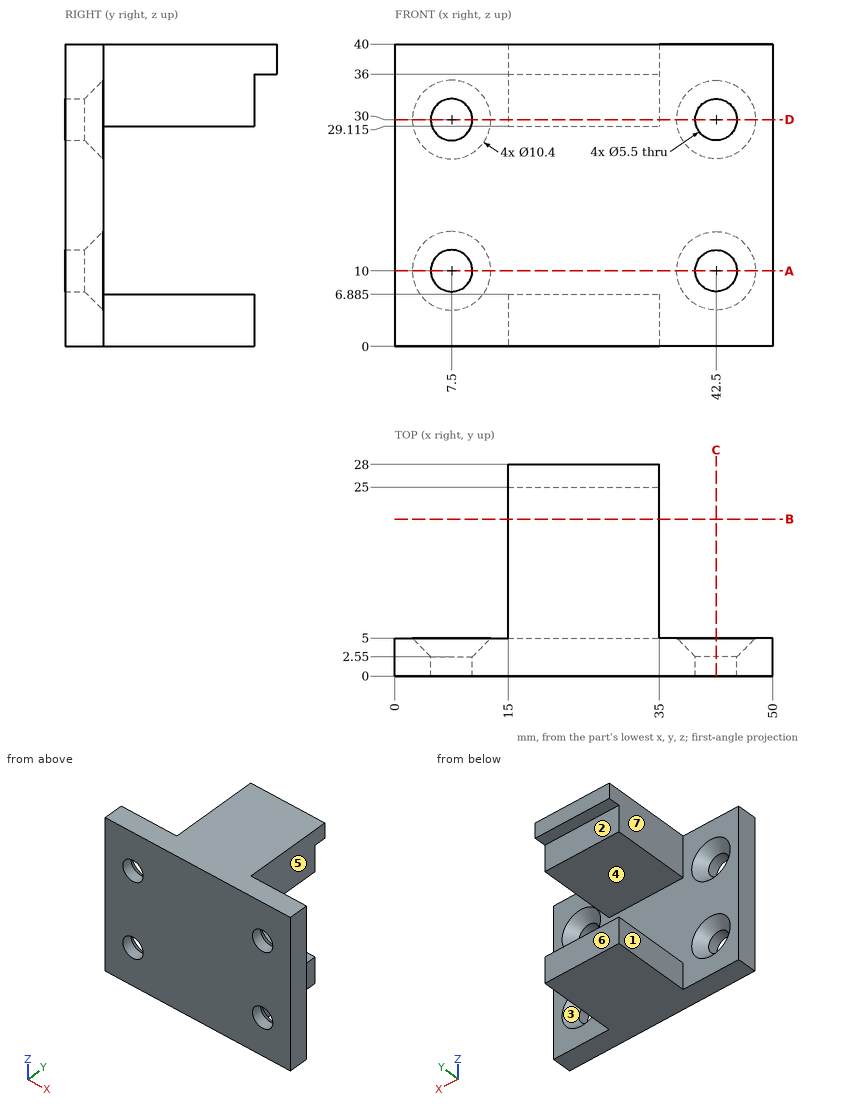
The figure shows three views and two pictorial views of one solid part (mm, origin at its lowest corner). Answer the questions. A direction names the side the tool comes from. Give positions to 0.01 mm unless a question says otherwise; leave off trailing zeros. Loops run counter-clockwise (first coordinate to the right, second up) from the corner with the lowest first, then second, coordinate; pieces in that order, holes last. Notation, with made-up numbers: (83.5, -16) -> (91.5, -16) arc R10 ccw to (91.5, -4) -> close; hole circle Ø8 at (40.5, 45.5). An arc over 180 degrees is marked (long way). Use a Markdown table: item, result. Add a question column.
1. Section C-C on x = 42.5 is taken. Determine the outline of the cut face in (y, z).
2. Section B-B on y = 20.75 is taken. Determine the outline of the cut face in (x, z) (3 decimals), and give its area (3 significant figures).
3. Find the intervals of material crossed by probe 1 along X at (y, z) = (1.45, 10); probe 2 along Z at (x, y) = (32, 14.5) (3 decimals); probe 3 along Z at (x, y) = (7.5, 1.4), in increasing order.
4. Section D-D on z = 30 is taken. Determine the outline of the cut face in (x, y), and give its area (3 significant figures).
5. Flat-ended cylindrical pins translate along their axes: pin 1 Ø10 at (x, y) = (9.5, 22) entering from -Z; pin 2 Ø7.5 at (y, z) = (16.5, 3.5) entering from -X; pin 3 Ø9 at (x, z) = (7.5, 30) entering from +Y; pin 4 Ø2 at (x, z) = (21, 31) entering from +Y. Find the tip coordinate at first contact, or state that the pin passes through.
6. For the marked faces 4, 5, 6 and 7, determine the directions among +Z, -Z, +X, -X, +Y, -Y from which every point of the face is accessible in a straight line to the end or side of a thin tool.
7. Determine the mould class of the marked faces 1, 2 and 3 for opening direction X: released by +X, released by -X, zero draft, split by the parting line, or undercut.
8. Section A-A on z = 10 is taken. Determine the outline of the cut face in (x, y), and give its area (3 significant figures).
Results below:
| question | item | result |
|---|---|---|
| 1 | outline | (0, 0) -> (5, 0) -> (5, 4.8) -> (2.55, 7.25) -> (0, 7.25) -> close; (0, 12.75) -> (2.55, 12.75) -> (5, 15.2) -> (5, 24.8) -> (2.55, 27.25) -> (0, 27.25) -> close; (0, 32.75) -> (2.55, 32.75) -> (5, 35.2) -> (5, 40) -> (0, 40) -> close |
| 2 | outline | (15, 0) -> (35, 0) -> (35, 6.885) -> (15, 6.885) -> close; (15, 29.115) -> (35, 29.115) -> (35, 40) -> (15, 40) -> close |
| 2 | area | 355 mm^2 |
| 3 | probe 1 | x = 0 to 4.75, 10.25 to 39.75, 45.25 to 50 |
| 3 | probe 2 | z = 0 to 6.885, 29.115 to 40 |
| 3 | probe 3 | z = 0 to 7.25, 12.75 to 27.25, 32.75 to 40 |
| 4 | outline | (0, 0) -> (4.75, 0) -> (4.75, 2.55) -> (2.3, 5) -> (0, 5) -> close; (10.25, 0) -> (39.75, 0) -> (39.75, 2.55) -> (37.3, 5) -> (35, 5) -> (35, 25) -> (15, 25) -> (15, 5) -> (12.7, 5) -> (10.25, 2.55) -> close; (45.25, 0) -> (50, 0) -> (50, 5) -> (47.7, 5) -> (45.25, 2.55) -> close |
| 4 | area | 583 mm^2 |
| 5 | pin 1 | passes through |
| 5 | pin 2 | stops at x = 15 |
| 5 | pin 3 | stops at y = 4.3 |
| 5 | pin 4 | stops at y = 25 |
| 6 | face 4 | +X, -X, +Y |
| 6 | face 5 | +Z, -Z, +X, +Y |
| 6 | face 6 | -Z, +X, -X, +Y |
| 6 | face 7 | +Z, -Z, -X, +Y |
| 7 | face 1 | released by -X |
| 7 | face 2 | zero draft |
| 7 | face 3 | undercut |
| 8 | outline | (0, 0) -> (4.75, 0) -> (4.75, 2.55) -> (2.3, 5) -> (0, 5) -> close; (10.25, 0) -> (39.75, 0) -> (39.75, 2.55) -> (37.3, 5) -> (12.7, 5) -> (10.25, 2.55) -> close; (45.25, 0) -> (50, 0) -> (50, 5) -> (47.7, 5) -> (45.25, 2.55) -> close |
| 8 | area | 183 mm^2 |
